Could you check a few things on this model? Use its own coordinates, in mm. Face numbers are marked on the shaded views. A direction names the side the tool comes from. Coordinates: 2 decimals unless noted, no trailing zeros. Loops run counter-clockwise (first coordinate to the right, second up) from the corner with the lowest first, then second, coordinate; pieces in that order, holes last. Notation, with made-up numbers: M 1.5,89.5 L 24.5,89.5 A26 ccw 24.5,124.5 Z; hole C -39,27 d9. An arc over 180 degrees is marked long. Return JSON: item names as keys, results as strings. Group by question number.
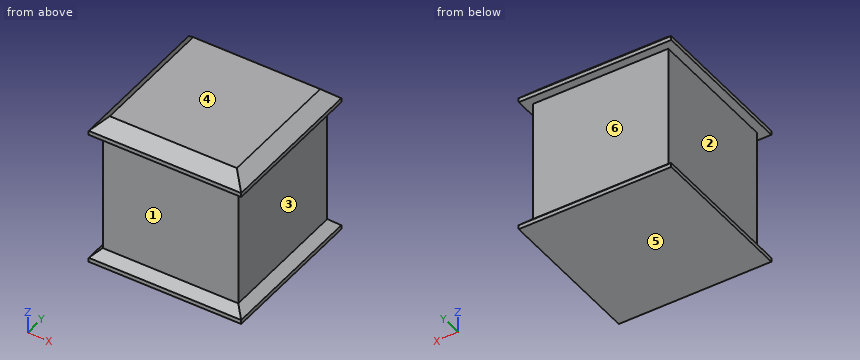
from build123d import *

# Parameters (mm, degrees)
F0_W          = 101.6
F0_H          = 6.35
F0_H_2        = 88.9
F1_DEPTH      = 50.8
F2_DEPTH      = 57.15
F3_DEPTH      = 57.15
F4_T1_DEPTH   = 163.2905609208
F4_T3_DEPTH   = 163.2905609208
F4_T8_DEPTH   = 163.2905609208
F4_T14_DEPTH  = 163.2905609208
F4_T20_DEPTH  = 163.2905609208
F4_T27_DEPTH  = 163.2905609208
F4_T33_DEPTH  = 163.2905609208
F4_T39_DEPTH  = 163.2905609208
F4_T45_DEPTH  = 163.2905609208
F4_T51_DEPTH  = 163.2905609208
F4_T58_DEPTH  = 163.2905609208
F4_T64_DEPTH  = 163.2905609208
F4_T70_DEPTH  = 163.2905609208
F4_T76_DEPTH  = 163.2905609208
F4_T82_DEPTH  = 163.2905609208
F4_T89_DEPTH  = 163.2905609208
F4_T95_DEPTH  = 163.2905609208
F4_T101_DEPTH = 163.2905609208
F4_T107_DEPTH = 163.2905609208
F4_T113_DEPTH = 163.2905609208
F4_T120_DEPTH = 163.2905609208
F4_T126_DEPTH = 163.2905609208


# Not quite as in the source:
# - a fillet or chamfer that OpenCascade refuses, or shapes differently, is made with other operations: its cross-section is extruded or revolved along the edge and cut away or added


with BuildPart() as f1:
    # F0 (on Front) → F1 (new body, symmetric)
    with BuildSketch(Plane.XZ):
        with Locations((0, -47.625)):
            Rectangle(F0_W, F0_H)
        Rectangle(F0_W, F0_H_2)
        with Locations((0, 47.625)):
            Rectangle(F0_W, F0_H)
    extrude(amount=F1_DEPTH, both=True)

    # F0 (on Front) → F2 (join, symmetric)
    with BuildSketch(Plane.XZ):
        Polygon((-50.8, 44.45), (-50.8, 50.8), (50.8, 50.8), (50.8, 44.45), (57.15, 44.45), (57.15, 57.15), (-57.15, 57.15), (-57.15, 44.45), align=None)
        Polygon((-50.8, -50.8), (-50.8, -44.45), (-57.15, -44.45), (-57.15, -57.15), (57.15, -57.15), (57.15, -44.45), (50.8, -44.45), (50.8, -50.8), align=None)
    extrude(amount=F2_DEPTH, both=True)

    # F0 (on Front) → F3 (join, symmetric)
    with BuildSketch(Plane.XZ):
        with Locations((0, 47.625)):
            Rectangle(F0_W, F0_H)
        with Locations((0, -47.625)):
            Rectangle(F0_W, F0_H)
    extrude(amount=F3_DEPTH, both=True)

    # F4: chamfer of 9.525 on 8 edges, made by hand

    # F4_s2 → F4_t1 (cut)
    with BuildSketch(Plane.YZ.offset(-81.6452804604)):
        Polygon((-47.625, 57.15), (-57.15, 47.625), (-57.15, 57.15), align=None)
        Polygon((47.625, 57.15), (57.15, 47.625), (57.15, 57.15), align=None)
    extrude(amount=F4_T1_DEPTH, mode=Mode.SUBTRACT)

    # F4_s4 → F4_t3 (cut)
    with BuildSketch(Plane.XZ.offset(-81.6452804604)):
        Polygon((47.625, 57.15), (57.15, 47.625), (57.15, 57.15), align=None)
        Polygon((-57.15, 47.625), (-47.625, 57.15), (-57.15, 57.15), align=None)
    extrude(amount=F4_T3_DEPTH, mode=Mode.SUBTRACT)


with BuildPart() as f4_tool6:
    # F4_s7 → F4_t8 (new body)
    with BuildSketch(Plane.XZ.offset(81.6452804604)):
        Polygon((47.625, -44.45), (57.15, -53.975), (57.15, -44.45), align=None)
    extrude(amount=-F4_T8_DEPTH)

    split(bisect_by=Plane.YZ.offset(50.8), keep=Keep.BOTTOM)

    split(bisect_by=Plane.XZ.offset(50.8), keep=Keep.TOP)


with BuildPart() as f1_1:
    add(f1.part)

    # F4_t5: cut F4_tool6
    add(f4_tool6.part, mode=Mode.SUBTRACT)


with BuildPart() as f4_tool12:
    # F4_s13 → F4_t14 (new body)
    with BuildSketch(Plane.XZ.offset(81.6452804604)):
        Polygon((47.625, -44.45), (57.15, -53.975), (57.15, -44.45), align=None)
    extrude(amount=-F4_T14_DEPTH)

    split(bisect_by=Plane.YZ.offset(50.8), keep=Keep.TOP)

    split(bisect_by=Plane.XZ.offset(50.8), keep=Keep.TOP)


with BuildPart() as f1_2:
    add(f1_1.part)

    # F4_t11: cut F4_tool12
    add(f4_tool12.part, mode=Mode.SUBTRACT)


with BuildPart() as f4_tool18:
    # F4_s19 → F4_t20 (new body)
    with BuildSketch(Plane.XZ.offset(81.6452804604)):
        Polygon((47.625, -44.45), (57.15, -53.975), (57.15, -44.45), align=None)
    extrude(amount=-F4_T20_DEPTH)

    split(bisect_by=Plane.XZ.offset(-50.8), keep=Keep.TOP)

    split(bisect_by=Plane.YZ.offset(50.8), keep=Keep.TOP)

    split(bisect_by=Plane.XZ.offset(50.8), keep=Keep.BOTTOM)


with BuildPart() as f1_3:
    add(f1_2.part)

    # F4_t17: cut F4_tool18
    add(f4_tool18.part, mode=Mode.SUBTRACT)


with BuildPart() as f4_tool25:
    # F4_s26 → F4_t27 (new body)
    with BuildSketch(Plane.XZ.offset(81.6452804604)):
        Polygon((47.625, -44.45), (57.15, -53.975), (57.15, -44.45), align=None)
    extrude(amount=-F4_T27_DEPTH)

    split(bisect_by=Plane.XZ.offset(-50.8), keep=Keep.BOTTOM)

    split(bisect_by=Plane.YZ.offset(50.8), keep=Keep.BOTTOM)


with BuildPart() as f1_4:
    add(f1_3.part)

    # F4_t24: cut F4_tool25
    add(f4_tool25.part, mode=Mode.SUBTRACT)


with BuildPart() as f4_tool31:
    # F4_s32 → F4_t33 (new body)
    with BuildSketch(Plane.XZ.offset(81.6452804604)):
        Polygon((47.625, -44.45), (57.15, -53.975), (57.15, -44.45), align=None)
    extrude(amount=-F4_T33_DEPTH)

    split(bisect_by=Plane.XZ.offset(-50.8), keep=Keep.BOTTOM)

    split(bisect_by=Plane.YZ.offset(50.8), keep=Keep.TOP)


with BuildPart() as f1_5:
    add(f1_4.part)

    # F4_t30: cut F4_tool31
    add(f4_tool31.part, mode=Mode.SUBTRACT)


with BuildPart() as f4_tool37:
    # F4_s38 → F4_t39 (new body)
    with BuildSketch(Plane.YZ.offset(-81.6452804604)):
        Polygon((-47.625, -44.45), (-57.15, -53.975), (-57.15, -44.45), align=None)
    extrude(amount=F4_T39_DEPTH)

    split(bisect_by=Plane.YZ.offset(-50.8), keep=Keep.BOTTOM)

    split(bisect_by=Plane.XZ.offset(50.8), keep=Keep.BOTTOM)


with BuildPart() as f1_6:
    add(f1_5.part)

    # F4_t36: cut F4_tool37
    add(f4_tool37.part, mode=Mode.SUBTRACT)


with BuildPart() as f4_tool43:
    # F4_s44 → F4_t45 (new body)
    with BuildSketch(Plane.YZ.offset(-81.6452804604)):
        Polygon((-47.625, -44.45), (-57.15, -53.975), (-57.15, -44.45), align=None)
    extrude(amount=F4_T45_DEPTH)

    split(bisect_by=Plane.YZ.offset(-50.8), keep=Keep.BOTTOM)

    split(bisect_by=Plane.XZ.offset(50.8), keep=Keep.TOP)


with BuildPart() as f1_7:
    add(f1_6.part)

    # F4_t42: cut F4_tool43
    add(f4_tool43.part, mode=Mode.SUBTRACT)


with BuildPart() as f4_tool49:
    # F4_s50 → F4_t51 (new body)
    with BuildSketch(Plane.YZ.offset(-81.6452804604)):
        Polygon((-47.625, -44.45), (-57.15, -53.975), (-57.15, -44.45), align=None)
    extrude(amount=F4_T51_DEPTH)

    split(bisect_by=Plane.YZ.offset(-50.8), keep=Keep.TOP)

    split(bisect_by=Plane.YZ.offset(50.8), keep=Keep.BOTTOM)

    split(bisect_by=Plane.XZ.offset(50.8), keep=Keep.TOP)


with BuildPart() as f1_8:
    add(f1_7.part)

    # F4_t48: cut F4_tool49
    add(f4_tool49.part, mode=Mode.SUBTRACT)


with BuildPart() as f4_tool56:
    # F4_s57 → F4_t58 (new body)
    with BuildSketch(Plane.YZ.offset(-81.6452804604)):
        Polygon((-47.625, -44.45), (-57.15, -53.975), (-57.15, -44.45), align=None)
    extrude(amount=F4_T58_DEPTH)

    split(bisect_by=Plane.YZ.offset(50.8), keep=Keep.TOP)

    split(bisect_by=Plane.XZ.offset(50.8), keep=Keep.BOTTOM)


with BuildPart() as f1_9:
    add(f1_8.part)

    # F4_t55: cut F4_tool56
    add(f4_tool56.part, mode=Mode.SUBTRACT)


with BuildPart() as f4_tool62:
    # F4_s63 → F4_t64 (new body)
    with BuildSketch(Plane.YZ.offset(-81.6452804604)):
        Polygon((-47.625, -44.45), (-57.15, -53.975), (-57.15, -44.45), align=None)
    extrude(amount=F4_T64_DEPTH)

    split(bisect_by=Plane.YZ.offset(50.8), keep=Keep.TOP)

    split(bisect_by=Plane.XZ.offset(50.8), keep=Keep.TOP)


with BuildPart() as f1_10:
    add(f1_9.part)

    # F4_t61: cut F4_tool62
    add(f4_tool62.part, mode=Mode.SUBTRACT)


with BuildPart() as f4_tool68:
    # F4_s69 → F4_t70 (new body)
    with BuildSketch(Plane.XZ.offset(-81.6452804604)):
        Polygon((-47.625, -44.45), (-57.15, -53.975), (-57.15, -44.45), align=None)
    extrude(amount=F4_T70_DEPTH)

    split(bisect_by=Plane.YZ.offset(-50.8), keep=Keep.TOP)

    split(bisect_by=Plane.XZ.offset(-50.8), keep=Keep.BOTTOM)


with BuildPart() as f1_11:
    add(f1_10.part)

    # F4_t67: cut F4_tool68
    add(f4_tool68.part, mode=Mode.SUBTRACT)


with BuildPart() as f4_tool74:
    # F4_s75 → F4_t76 (new body)
    with BuildSketch(Plane.XZ.offset(-81.6452804604)):
        Polygon((-47.625, -44.45), (-57.15, -53.975), (-57.15, -44.45), align=None)
    extrude(amount=F4_T76_DEPTH)

    split(bisect_by=Plane.YZ.offset(-50.8), keep=Keep.BOTTOM)

    split(bisect_by=Plane.XZ.offset(-50.8), keep=Keep.BOTTOM)


with BuildPart() as f1_12:
    add(f1_11.part)

    # F4_t73: cut F4_tool74
    add(f4_tool74.part, mode=Mode.SUBTRACT)


with BuildPart() as f4_tool80:
    # F4_s81 → F4_t82 (new body)
    with BuildSketch(Plane.XZ.offset(-81.6452804604)):
        Polygon((-47.625, -44.45), (-57.15, -53.975), (-57.15, -44.45), align=None)
    extrude(amount=F4_T82_DEPTH)

    split(bisect_by=Plane.YZ.offset(-50.8), keep=Keep.BOTTOM)

    split(bisect_by=Plane.XZ.offset(-50.8), keep=Keep.TOP)

    split(bisect_by=Plane.XZ.offset(50.8), keep=Keep.BOTTOM)


with BuildPart() as f1_13:
    add(f1_12.part)

    # F4_t79: cut F4_tool80
    add(f4_tool80.part, mode=Mode.SUBTRACT)


with BuildPart() as f4_tool87:
    # F4_s88 → F4_t89 (new body)
    with BuildSketch(Plane.XZ.offset(-81.6452804604)):
        Polygon((-47.625, -44.45), (-57.15, -53.975), (-57.15, -44.45), align=None)
    extrude(amount=F4_T89_DEPTH)

    split(bisect_by=Plane.YZ.offset(-50.8), keep=Keep.TOP)

    split(bisect_by=Plane.XZ.offset(50.8), keep=Keep.TOP)


with BuildPart() as f1_14:
    add(f1_13.part)

    # F4_t86: cut F4_tool87
    add(f4_tool87.part, mode=Mode.SUBTRACT)


with BuildPart() as f4_tool93:
    # F4_s94 → F4_t95 (new body)
    with BuildSketch(Plane.XZ.offset(-81.6452804604)):
        Polygon((-47.625, -44.45), (-57.15, -53.975), (-57.15, -44.45), align=None)
    extrude(amount=F4_T95_DEPTH)

    split(bisect_by=Plane.YZ.offset(-50.8), keep=Keep.BOTTOM)

    split(bisect_by=Plane.XZ.offset(50.8), keep=Keep.TOP)


with BuildPart() as f1_15:
    add(f1_14.part)

    # F4_t92: cut F4_tool93
    add(f4_tool93.part, mode=Mode.SUBTRACT)


with BuildPart() as f4_tool99:
    # F4_s100 → F4_t101 (new body)
    with BuildSketch(Plane.YZ.offset(81.6452804604)):
        Polygon((47.625, -44.45), (57.15, -53.975), (57.15, -44.45), align=None)
    extrude(amount=-F4_T101_DEPTH)

    split(bisect_by=Plane.XZ.offset(-50.8), keep=Keep.TOP)

    split(bisect_by=Plane.YZ.offset(50.8), keep=Keep.TOP)


with BuildPart() as f1_16:
    add(f1_15.part)

    # F4_t98: cut F4_tool99
    add(f4_tool99.part, mode=Mode.SUBTRACT)


with BuildPart() as f4_tool105:
    # F4_s106 → F4_t107 (new body)
    with BuildSketch(Plane.YZ.offset(81.6452804604)):
        Polygon((47.625, -44.45), (57.15, -53.975), (57.15, -44.45), align=None)
    extrude(amount=-F4_T107_DEPTH)

    split(bisect_by=Plane.XZ.offset(-50.8), keep=Keep.BOTTOM)

    split(bisect_by=Plane.YZ.offset(50.8), keep=Keep.TOP)


with BuildPart() as f1_17:
    add(f1_16.part)

    # F4_t104: cut F4_tool105
    add(f4_tool105.part, mode=Mode.SUBTRACT)


with BuildPart() as f4_tool111:
    # F4_s112 → F4_t113 (new body)
    with BuildSketch(Plane.YZ.offset(81.6452804604)):
        Polygon((47.625, -44.45), (57.15, -53.975), (57.15, -44.45), align=None)
    extrude(amount=-F4_T113_DEPTH)

    split(bisect_by=Plane.YZ.offset(-50.8), keep=Keep.TOP)

    split(bisect_by=Plane.XZ.offset(-50.8), keep=Keep.BOTTOM)

    split(bisect_by=Plane.YZ.offset(50.8), keep=Keep.BOTTOM)


with BuildPart() as f1_18:
    add(f1_17.part)

    # F4_t110: cut F4_tool111
    add(f4_tool111.part, mode=Mode.SUBTRACT)


with BuildPart() as f4_tool118:
    # F4_s119 → F4_t120 (new body)
    with BuildSketch(Plane.YZ.offset(81.6452804604)):
        Polygon((47.625, -44.45), (57.15, -53.975), (57.15, -44.45), align=None)
    extrude(amount=-F4_T120_DEPTH)

    split(bisect_by=Plane.YZ.offset(-50.8), keep=Keep.BOTTOM)

    split(bisect_by=Plane.XZ.offset(-50.8), keep=Keep.TOP)


with BuildPart() as f1_19:
    add(f1_18.part)

    # F4_t117: cut F4_tool118
    add(f4_tool118.part, mode=Mode.SUBTRACT)


with BuildPart() as f4_tool124:
    # F4_s125 → F4_t126 (new body)
    with BuildSketch(Plane.YZ.offset(81.6452804604)):
        Polygon((47.625, -44.45), (57.15, -53.975), (57.15, -44.45), align=None)
    extrude(amount=-F4_T126_DEPTH)

    split(bisect_by=Plane.YZ.offset(-50.8), keep=Keep.BOTTOM)

    split(bisect_by=Plane.XZ.offset(-50.8), keep=Keep.BOTTOM)


with BuildPart() as f1_20:
    add(f1_19.part)

    # F4_t123: cut F4_tool124
    add(f4_tool124.part, mode=Mode.SUBTRACT)


solid = f1_20.part
(1) If I drill on L1, parallel to X at y = 35.5, z = -25; L2, parallel to Y at x = 47, z = 50 (3 decimals), over which ranges is the centre line in solid material (lowest first)? Write a range as [from, to].
(2) Imagine slicing it at A-A, the plane x = 44.5. Write out the boundary of the cut face in (y, z) (3 decimals), then the cut area to 3 significant figures.
(3) Imagine slicing it at C-C, the plane z = 23. Write out the boundary of the cut face in (x, y).
(4) Will these pins go through, and if not, where does the flat tip stop? P1, Ø3, axis at y = 10.5, z = 26, coming from the +X side; P2, Ø2, axis at x = 16, z = -24.5, coming from the +Y side; P3, Ø8, axis at y = 35, z = -44, coming from the +X side (3 decimals).
(5) For the marked faces 1, 2 and 3, which set-ups out of +Z, -Z, +X, -X, +Y, -Y let a thin tool reach every point of the face, with its end or its side?
(6) We'd pull the mould along Z, two halves only. Please class the marked faces 4, 5 and 6: +Z half, -Z half, draft (parallel to the pull), parting line (faces both ways), or undercut.
Checks:
{
 "1": {"L1": "[-50.8, 50.8]", "L2": "[-54.775, 54.775]"},
 "2": {"outline": "M -57.15,-57.15 L 57.15,-57.15 L 57.15,-53.975 L 50.8,-47.625 L 50.8,44.45 L 57.15,44.45 L 57.15,47.625 L 47.625,57.15 L -47.625,57.15 L -57.15,47.625 L -57.15,44.45 L -50.8,44.45 L -50.8,-47.625 L -57.15,-53.975 Z", "area": "11,800 mm²"},
 "3": {"outline": "M -50.8,-50.8 L 50.8,-50.8 L 50.8,50.8 L -50.8,50.8 Z"},
 "4": {"P1": "x = 50.8", "P2": "y = 50.8", "P3": "x = 51.175"},
 "5": {"face 1": "+X, -X, -Y", "face 2": "-X, +Y, -Y", "face 3": "+X, +Y, -Y"},
 "6": {"face 4": "+Z half", "face 5": "-Z half", "face 6": "undercut"}
}
